CAD build for the part. Positions are in the model's coordinates, mm. A direction names the side the tool comes from. Round coordinates to 2 decimals unless told otherwise and drop trailing zeros. Loops run counter-clockwise (first coordinate to the right, second up) from the corner with the lowest first, then second, coordinate; pieces in that order, holes last. Notation, with made-up numbers: M 23.5,44 L 27.5,44 A22 cw 27.5,60 Z; hole C 34,85 d5. An arc over 180 degrees is marked long. Put each result on its own line as item: value. Start each with the question number.
from build123d import *

# Parameters (mm, degrees)
BOSS_EXTRUDE1_DEPTH  = 7
CUT_EXTRUDE1_DEPTH   = 0.2
FILLET1_R            = 2.5
CHAMFER1_SIZE        = 6
CUT_EXTRUDE4_DEPTH   = 2.2
CUT_EXTRUDE5_DEPTH   = 59.720013624
SKETCH14_R           = 2.2
CUT_EXTRUDE9_DEPTH   = 0.2
CUT_EXTRUDE10_DEPTH  = 4.11
CHAMFER3_SIZE        = 1
FILLET3_R            = 3.2
SKETCH29_R           = 1.05
CUT_EXTRUDE16_DEPTH  = 10
FILLET5_R            = 2
FILLET6_R            = 2
MIRROR2_COPY_1_DEPTH = 2.2
SKETCH31_R           = 1.75
CUT_EXTRUDE17_DEPTH  = 0.5
CUT_EXTRUDE19_START  = -4.1
CUT_EXTRUDE19_DEPTH  = 4.1
SKETCH33_R           = 2.1
BOSS_EXTRUDE2_DEPTH  = 10


with BuildPart() as part:
    # Sketch1 → Boss-Extrude1 (new body)
    with BuildSketch(Plane.XY):
        with BuildLine():
            Line((0, -4), (0, 17))
            Line((0, 17), (56, 17))
            Line((56, 17), (56, -4))
            ThreePointArc((56, -4), (54.974873734, -6.474873734), (52.5, -7.5))
            Line((52.5, -7.5), (36.5, -7.5))
            Line((36.5, -7.5), (36.5, -11.4))
            Line((36.5, -11.4), (19.5, -11.4))
            Line((19.5, -11.4), (19.5, -7.5))
            Line((19.5, -7.5), (3.5, -7.5))
            ThreePointArc((3.5, -7.5), (1.025126266, -6.474873734), (0, -4))
        make_face()
    extrude(amount=BOSS_EXTRUDE1_DEPTH)

    # Sketch2 → Cut-Extrude1 (cut)
    with BuildSketch(Plane.XY.offset(7)):
        Polygon((5, 15.8), (5, 0.8), (50.15, 0.8), (53.15, 3.8), (53.15, 9.9), (47.25, 15.8), align=None)
    extrude(amount=-CUT_EXTRUDE1_DEPTH, mode=Mode.SUBTRACT)

    # Fillet1
    fillet1_edges = [part.edges().sort_by_distance(p)[0] for p in [
        (47.25, 15.8, 6.9),
        (53.15, 9.9, 6.9),
        (53.15, 3.8, 6.9),
        (50.15, 0.8, 6.9),
        (5, 0.8, 6.9),
        (5, 15.8, 6.9),
    ]]
    fillet(fillet1_edges, radius=FILLET1_R)

    # Chamfer1
    chamfer1_edges = [part.edges().sort_by_distance(p)[0] for p in [
        (56, 17, 3.5),
    ]]
    chamfer(chamfer1_edges, length=CHAMFER1_SIZE)

    # Sketch6 → Cut-Extrude4 (cut)
    with BuildSketch(Plane.XY.offset(7)):
        with BuildLine():
            Line((49.7, -4), (49.7, -2))
            ThreePointArc((49.7, -2), (52.5, 0.8), (55.3, -2))
            Line((55.3, -2), (55.3, -4))
            ThreePointArc((55.3, -4), (52.5, -6.8), (49.7, -4))
        make_face()
    cut_extrude4 = extrude(amount=-CUT_EXTRUDE4_DEPTH, mode=Mode.SUBTRACT)

    # Sketch9 → Cut-Extrude5 (cut, through all)
    with BuildSketch(Plane.XY.offset(4.8)):
        with BuildLine():
            Line((54.15, -4), (54.15, -2))
            ThreePointArc((54.15, -2), (52.5, -0.35), (50.85, -2))
            Line((50.85, -2), (50.85, -4))
            ThreePointArc((50.85, -4), (52.5, -5.65), (54.15, -4))
        make_face()
    cut_extrude5 = extrude(amount=-CUT_EXTRUDE5_DEPTH, mode=Mode.SUBTRACT)

    # Mirror1: Cut-Extrude4 across plane
    add(cut_extrude4.mirror(Plane.XY.offset(3.5)), mode=Mode.SUBTRACT)

    # Sketch14 → Cut-Extrude9 (cut)
    with BuildSketch(Plane(origin=(0, 24, 0), x_dir=(0, -1, 0), z_dir=(1, 0, 0))):
        with Locations(Location((16, -3.5, 0), (0, 0, 90))):
            Circle(SKETCH14_R)
    extrude(amount=CUT_EXTRUDE9_DEPTH, mode=Mode.SUBTRACT)

    # Sketch19 → Cut-Extrude10 (cut)
    with BuildSketch(Plane.XY.offset(7)):
        with BuildLine():
            Line((20.8, -0.4), (35.2, -0.4))
            Line((35.2, -0.4), (35.2, -8.2))
            ThreePointArc((35.2, -8.2), (34.614213562, -9.614213562), (33.2, -10.2))
            Line((33.2, -10.2), (22.8, -10.2))
            ThreePointArc((22.8, -10.2), (21.385786438, -9.614213562), (20.8, -8.2))
            Line((20.8, -8.2), (20.8, -0.4))
        make_face()
    extrude(amount=-CUT_EXTRUDE10_DEPTH, mode=Mode.SUBTRACT)

    # Chamfer3
    chamfer3_edges = [part.edges().sort_by_distance(p)[0] for p in [
        (0, 17, 3.5),
    ]]
    chamfer(chamfer3_edges, length=CHAMFER3_SIZE)

    # Fillet3
    fillet3_edges = [part.edges().sort_by_distance(p)[0] for p in [
        (36.5, -11.4, 3.5),
        (19.5, -11.4, 3.5),
    ]]
    fillet(fillet3_edges, radius=FILLET3_R)

    # Sketch29 → Cut-Extrude16 (cut)
    with BuildSketch(Plane(origin=(0, 0, 0), x_dir=(-1, 0, 0), z_dir=(0, 0, -1))):
        with Locations((-42.65, -5.5)):
            Circle(SKETCH29_R)
        with Locations((-41, -2.7)):
            Circle(SKETCH29_R)
        with Locations((-13.35, -5.5)):
            Circle(SKETCH29_R)
        with Locations((-15, -2.7)):
            Circle(SKETCH29_R)
    extrude(amount=-CUT_EXTRUDE16_DEPTH, mode=Mode.SUBTRACT)

    # Fillet5
    # the kernel refuses this fillet: 2 mm, written as the material it adds along each edge
    with BuildSketch(Plane(origin=(19.5, -7.5, 0), x_dir=(0.06758731351152399, -0.9977133631721562, 0), z_dir=(0, 0, 1))) as fillet5_piece_1:
        with BuildLine():
            CenterArc((1.871412228, -1.965857277), FILLET5_R, 100.602090028, 75.522487814)
            Line((-0.124014498, -1.83068265), (-0.323557171, -1.817165187))
            Line((-0.323557171, -1.817165187), (-0.199542673, 0.013517463))
            Line((-0.199542673, 0.013517463), (0.013517463, 0.199542673))
            ThreePointArc((0.013517463, 0.199542673), (0.711916817, 0.152231553), (1.466640375, 0.196585728))
            Line((1.466640375, 0.196585728), (1.503437816, 0))
        make_face()
    extrude(amount=7)
    # the kernel refuses this fillet: 2 mm, written as the material it takes off along each edge

    # Fillet6
    # the kernel refuses this fillet: 2 mm, written as the material it adds along each edge
    with BuildSketch(Plane(origin=(36.5, -7.5, 0), x_dir=(-0.06758731351152392, -0.9977133631721562, 0), z_dir=(0, 0, 1))) as fillet6_piece_1:
        with BuildLine():
            CenterArc((1.871412228, 1.965857277), FILLET6_R, 183.875422158, 75.522487814)
            Line((-0.124014498, 1.83068265), (-0.323557171, 1.817165187))
            Line((-0.323557171, 1.817165187), (-0.199542673, -0.013517463))
            Line((-0.199542673, -0.013517463), (0.013517463, -0.199542673))
            ThreePointArc((0.013517463, -0.199542673), (0.711916817, -0.152231553), (1.466640375, -0.196585728))
            Line((1.466640375, -0.196585728), (1.503437816, 0))
        make_face()
    extrude(amount=7)
    # the kernel refuses this fillet: 2 mm, written as the material it takes off along each edge

    # Mirror2: Cut-Extrude4, Cut-Extrude5 across plane
    add(cut_extrude4.mirror(Plane.ZY.offset(-28)), mode=Mode.SUBTRACT)
    add(cut_extrude5.mirror(Plane.ZY.offset(-28)), mode=Mode.SUBTRACT)

    # Mirror2 copy 1 sketch → Mirror2 copy 1 (cut)
    with BuildSketch(Plane(origin=(56, 0, 0), x_dir=(-1, 0, 0), z_dir=(0, 0, -1))):
        with BuildLine():
            Line((49.7, -4), (49.7, -2))
            ThreePointArc((49.7, -2), (52.5, 0.8), (55.3, -2))
            Line((55.3, -2), (55.3, -4))
            ThreePointArc((55.3, -4), (52.5, -6.8), (49.7, -4))
        make_face()
    extrude(amount=-MIRROR2_COPY_1_DEPTH, mode=Mode.SUBTRACT)

    # Sketch31 → Cut-Extrude17 (cut)
    with BuildSketch(Plane.XY.offset(7)):
        with Locations((2.5, 8)):
            Circle(SKETCH31_R)
    extrude(amount=-CUT_EXTRUDE17_DEPTH, mode=Mode.SUBTRACT)

    # Sketch28 → Cut-Extrude19 (cut)
    with BuildSketch(Plane.XY.offset(7).offset(CUT_EXTRUDE19_START)):
        with BuildLine():
            Line((16.098076211, -0.767949192), (5.25, -7.031088913))
            ThreePointArc((5.25, -7.031088913), (4.405866658, -7.380740392), (3.5, -7.5))
            Line((3.5, -7.5), (16.682429586, -7.5))
            ThreePointArc((16.682429586, -7.5), (17.389536367, -7.792893219), (17.682429586, -8.5))
            Line((17.682429586, -8.5), (17.682429586, -14.577281055))
            Line((17.682429586, -14.577281055), (38.317570414, -14.577281055))
            Line((38.317570414, -14.577281055), (38.317570414, -8.5))
            ThreePointArc((38.317570414, -8.5), (38.610463633, -7.792893219), (39.317570414, -7.5))
            Line((39.317570414, -7.5), (52.5, -7.5))
            ThreePointArc((52.5, -7.5), (51.594133342, -7.380740392), (50.75, -7.031088913))
            Line((50.75, -7.031088913), (39.901923789, -0.767949192))
            ThreePointArc((39.901923789, -0.767949192), (39.419561879, -0.568148347), (38.901923789, -0.5))
            Line((38.901923789, -0.5), (37.5, -0.5))
            Line((37.5, -0.5), (37.5, -0.4))
            Line((37.5, -0.4), (18.5, -0.4))
            Line((18.5, -0.4), (18.5, -0.5))
            Line((18.5, -0.5), (17.098076211, -0.5))
            ThreePointArc((17.098076211, -0.5), (16.580438121, -0.568148347), (16.098076211, -0.767949192))
        make_face()
    extrude(amount=CUT_EXTRUDE19_DEPTH, mode=Mode.SUBTRACT)

    # Sketch32 → Revolve1 (revolve)
    with BuildSketch(Plane(origin=(0, 0, 3.8), x_dir=(-1, 0, 0), z_dir=(0, 0, -1))):
        with BuildLine():
            Line((-52.333452378, 14.666547622), (-53.464823228, 13.535176772))
            ThreePointArc((-53.464823228, 13.535176772), (-53.933452378, 14.666547622), (-53.464823228, 15.797918472))
            Line((-53.464823228, 15.797918472), (-52.333452378, 14.666547622))
        make_face()
    revolve(axis=Axis((52.333452378, 14.666547622, 3.8), (0.7071067811865478, 0.7071067811865472, 0)))

    # Sketch33 → Boss-Extrude2 (add)
    with BuildSketch(Plane.ZY.offset(-0.2)):
        with Locations(Location((3.5, 8, 0), (0, 0, 180))):
            Circle(SKETCH33_R)
    extrude(amount=BOSS_EXTRUDE2_DEPTH)


solid = part.part
(1) Drill centre lines: line 1 along Y through (x, z) = (41, 1.25); line 2 along Y through (x, z) = (13.35, 1.9); line 3 along X through (y, z) = (-0.25, 2). Where is each one in solid material? Low to high.
(2) Tool access for faces 4 (the flat face through (54.15, -3, 4)), 5 (the cylindrical face through (52.6, -6.8, 5.9)), 6 (the cylindrical face through (52.4, 0.8, 1.1)), 7 (the flat face through (27.8, 0.5, 7)), 8 (the flat face through (46, -7.5, 1)): list every direction of +Z, -Z, +X, -X, +Y, -Y with a clear straight run to the whole face (end or side of a thin tool).
(3) Cut at A-A on y = 8. List the corners of the cut face in (x, z).
(4) Mould opens along X. For faces 1 (the cylindrical face through (43.7, -5.5, 1.4)), 2 (the flat face through (-9.8, 8, 4)), 3 (the cylindrical face through (37.12, -7.91, 1.43)) say: +X half, -X half, draft (parallel to the pull), parting line (faces both ways), or undercut.
(5) Flat gauge pins, fed straight in: pin 1 Ø1 at (x, y) = (2.5, 7.5) entering from +Z; pin 2 Ø2.5 at (x, z) = (11.5, 1) entering from -Y; pin 3 Ø5 at (x, y) = (32.5, 7.5) entering from +Z. Where does each tip first touch, or does it go through?
(6) Cut at B-B on x = 15. List the corners of the cut face in (y, z).
Taken from the geometry:
1. line 1: -7.5 to -3.75, -1.65 to 17
1. line 2: -7.5 to -6.55, -4.45 to 17
1. line 3: 0 to 1.31, 5.69 to 50.31, 54.69 to 56
2. face 4: +Z, -Z
2. face 5: +Z
2. face 6: -Z
2. face 7: +Z, +X, -X, +Y, -Y
2. face 8: +Z, -Z, +X, -Y
3. outline: M -9.8,1.4 L 0.2,1.4 L 0.2,1.3 L 0,1.3 L 0,0 L 56,0 L 56,7 L 53.15,7 L 53.15,6.8 L 5,6.8 L 5,7 L 4.25,7 L 4.25,6.5 L 0.75,6.5 L 0.75,7 L 0,7 L 0,5.7 L 0.2,5.7 L 0.2,5.6 L -9.8,5.6 Z
4. face 1: undercut
4. face 2: -X half
4. face 3: +X half
5. pin 1: z = 6.5
5. pin 2: y = -7.5
5. pin 3: z = 6.8
6. outline: M -7.5,0 L -3.75,0 L -3.75,2.9 L -7.5,2.9 Z; M -1.65,0 L 17,0 L 17,7 L 15.8,7 L 15.8,6.8 L 0.8,6.8 L 0.8,7 L -1.4,7 L -1.4,2.9 L -1.65,2.9 Z
